Geometry: final body of the model. Coordinates: model frame, mm. Face numbers are marked on the shaded views. A direction names the side the tool comes from. Give positions to 0.01 mm unless a question says otherwise; leave off trailing zeros. Loops run counter-clockwise (first coordinate to the right, second up) from the corner with the lowest first, then second, coordinate; pieces in that order, holes last.
1. Material intervals for line 1 along Z through (x, y) = (66, -710); line 2 along Z through (x, y) = (61.5, -706); line 3 along Z through (x, y) = (13, -730), sorted ascending.
2. Draft query along Z for the marked faces 6, 7 and 8. Return one class per face: +Z half, -Z half, draft (parallel to the pull), parting line (faces both ways), or undercut.
3. Access query for the marked faces 1, 2, 3, 4 and 5. Directions: +Z, -Z, +X, -X, +Y, -Y. A direction counts if a zero-diameter tool reaches every point of the face in a straight line with its end or side. Return the directions, or none.
4. Section A-A, the plane y = -710. Output: boundary loops of the cut face in (x, z).
5. First-contact query: P1, Ø1, axis at x = 30.5, z = -410, coming from the -Y side; P2, Ø6, axis at x = 48.5, y = -733, coming from the +Z side; P3, Ø17, axis at x = 30, z = -157, coming from the +Y side. Flat tips, straight axial feed; report the tip coordinate or a pass-through.
6. Section B-B, the plane z = -254.5. Output: boundary loops of the cut face in (x, y).
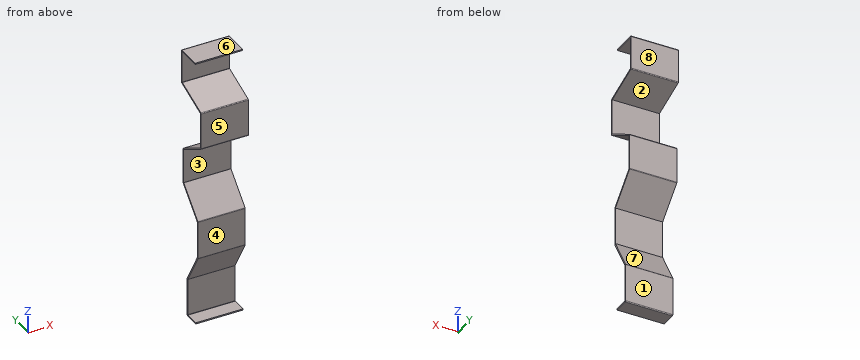
from build123d import *

# Parameters (mm, degrees)
BOSS_EXTRUDE1_DEPTH = 76.2
FILLET1_R           = 1.5
FILLET2_R           = 1.5
FILLET3_R           = 0.5


with BuildPart() as part:
    # Sketch1 → Boss-Extrude1 (new body)
    with BuildSketch(Plane(origin=(0, 0, 0), x_dir=(0, 0, -1), z_dir=(1, 0, 0))):
        Polygon((410.975974775, -727.738016425), (410.975974775, -702.338016425), (347.983974775, -702.338016425), (296.022450548, -732.338016425), (236.022450548, -732.338016425), (193.596043677, -689.911609554), (135.596043677, -689.911609554), (105.596043677, -741.873133781), (47.596043677, -741.873133781), (27.074835078, -685.491576534), (-28.635164922, -685.491576534), (-28.635164922, -726.131576534), (-26.635164922, -726.131576534), (-26.635164922, -687.491576534), (25.566835078, -687.491576534), (46.088043677, -743.873133781), (106.588043677, -743.873133781), (136.588043677, -691.911609554), (192.588043677, -691.911609554), (235.014450548, -734.338016425), (297.014450548, -734.338016425), (348.975974775, -704.338016425), (408.975974775, -704.338016425), (408.975974775, -727.738016425), align=None)
    extrude(amount=BOSS_EXTRUDE1_DEPTH)

    # Fillet1
    fillet1_edges = [part.edges().sort_by_distance(p)[0] for p in [
        (38.1, -685.491576534, 28.635164922),
        (38.1, -685.491576534, -27.074835078),
        (38.1, -689.911609554, -135.596043677),
        (38.1, -689.911609554, -193.596043677),
        (38.1, -702.338016425, -347.983974775),
        (38.1, -702.338016425, -410.975974775),
    ]]
    fillet(fillet1_edges, radius=FILLET1_R)

    # Fillet2
    fillet2_edges = [part.edges().sort_by_distance(p)[0] for p in [
        (38.1, -734.338016425, -297.014450548),
        (38.1, -734.338016425, -235.014450548),
        (38.1, -743.873133781, -106.588043677),
        (38.1, -743.873133781, -46.088043677),
    ]]
    fillet(fillet2_edges, radius=FILLET2_R)

    # Fillet3
    fillet3_edges = [part.edges().sort_by_distance(p)[0] for p in [
        (38.1, -704.338016425, -408.975974775),
        (38.1, -704.338016425, -348.975974775),
        (38.1, -691.911609554, -192.588043677),
        (38.1, -691.911609554, -136.588043677),
        (38.1, -687.491576534, -25.566835078),
        (38.1, -687.491576534, 26.635164922),
    ]]
    fillet(fillet3_edges, radius=FILLET3_R)


solid = part.part
Answers below:
1. line 1: z = -410.98 to -408.98, -339.17 to -334.71, -213.68 to -210.68, -126.14 to -124, -36 to -33.76, 26.64 to 28.64
1. line 2: z = -410.98 to -408.98, -346.1 to -341.64, -209.68 to -206.68, -128.45 to -126.31, -34.54 to -32.3, 26.64 to 28.64
1. line 3: z = -304.53 to -300.07, -233.68 to -230.68, -114.6 to -112.45, -43.27 to -41.04
2. face 6: +Z half
2. face 7: undercut
2. face 8: draft
3. face 1: -Z, +X, -X, +Y
3. face 2: +X, -X, +Y
3. face 3: +X, -X, -Y
3. face 4: -Z, +X, -X, -Y
3. face 5: +Z, -Z, +X, -X, -Y
4. outline: (0, -410.98) - (76.2, -410.98) - (76.2, -408.98) - (0, -408.98) - close; (0, -339.17) - (76.2, -339.17) - (76.2, -334.71) - (0, -334.71) - close; (0, -213.68) - (76.2, -213.68) - (76.2, -210.68) - (0, -210.68) - close; (0, -126.14) - (76.2, -126.14) - (76.2, -124) - (0, -124) - close; (0, -36) - (76.2, -36) - (76.2, -33.76) - (0, -33.76) - close; (0, 26.64) - (76.2, 26.64) - (76.2, 28.64) - (0, 28.64) - close
5. P1: stops at y = -727.74
5. P2: stops at z = -41.04
5. P3: stops at y = -689.91
6. outline: (0, -734.34) - (76.2, -734.34) - (76.2, -732.34) - (0, -732.34) - close
